Check sheet for the drawn part. Datum: minimum x, y, z corner. Units: mm. A direction names the side the tool comes from. Give positions to 0.01 mm unless a question says otherwise; leave off trailing zeros. Order: outer loops, then holes, each group sorted by start corner. A loop starts at its lowest first (then second) coordinate and runs counter-clockwise, first axis right, second up. Notation, with made-up numbers: M 23,60 L 73,60 A24 ccw 73,73 Z; hole C 14.5,-32 d4. An arc over 180 degrees is marked long. Answer as CSV lines item,"result". Start each with the question number.
Q1. Section check A-A, the plane x = 36. Record the boundary of the cut face in (y, z), then the cut area to 3 significant figures.
Q2. Go/stop test with flat-tipped pins: pin 1 (5 mm diameter, centred on x = 14.5, y = 16.5, fed in from -Z); pin 2 (4 mm diameter, centred on x = 26, z = 2, fed in from +Y); pin 3 (8 mm diameter, centred on x = 38, y = 40, fed in from -Z); pin 4 (6 mm diameter, centred on y = 15.5, z = 26, fed in from -X). Record where each tip stops, or that it passes through.
Q3. Set-up check for the marked faces 1, 2, 3, 4 and 5: record each of +Z, -Z, +X, -X, +Y, -Y from which the full face is reachable in a straight line by a thin tool's end or side.
Q4. Section check C-C, the plane y = 25. Record the boundary of the cut face in (x, z).
Q5. Mould release check, pull along Z, two halves, no side actions. Record for the marked faces 6, 7, 8 and 9: +Z half, -Z half, draft (parallel to the pull), parting line (faces both ways), or undercut.
Q6. Thickness scan on line 1 (X direction, y = 5.75, z = 23); line 2 (Y direction, x = 36, z = 10); line 3 (X direction, y = 42.5, z = 17). Record the ranges inside material, lowest first.
Q7. Section check B-B, the plane z = 22. Record the boundary of the cut face in (x, y).
Q8. Section check D-D, the plane z = 15. Record the boundary of the cut face in (x, y), then the cut area to 3 significant figures.
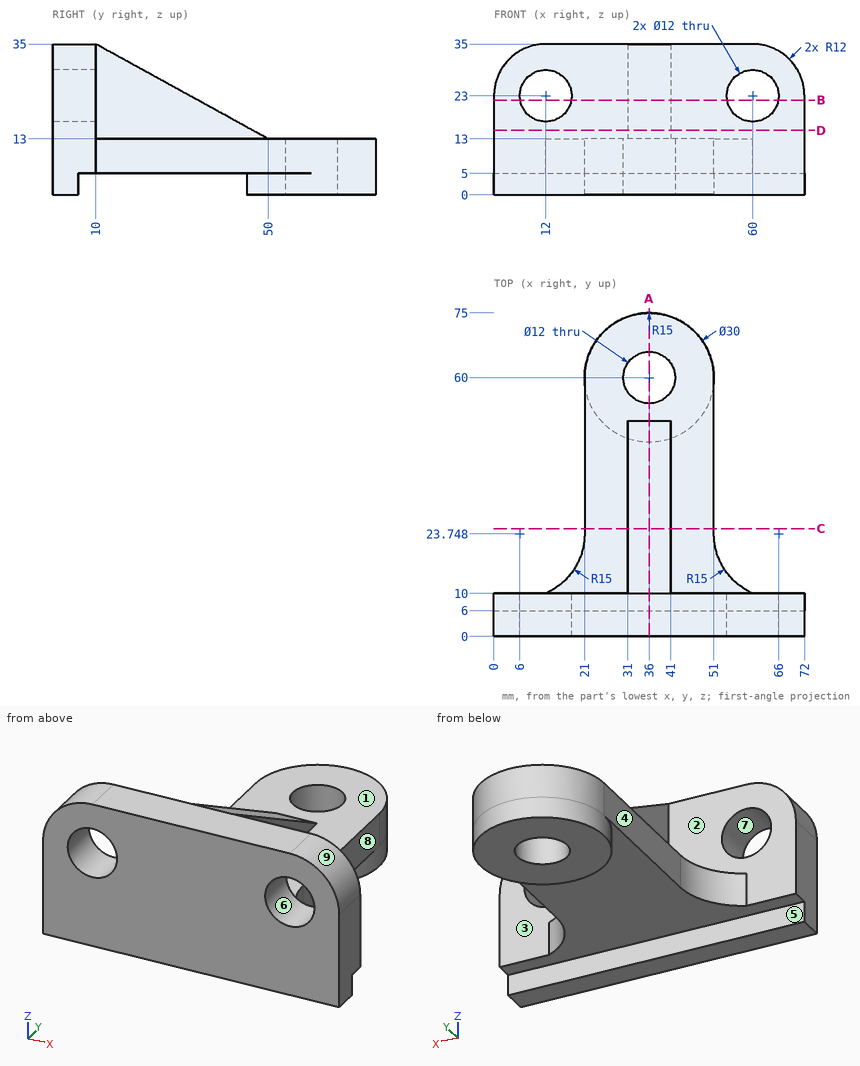
Answer block:
1,outline,"M 0,0 L 6,0 L 6,5 L 45,5 L 45,0 L 54,0 L 54,13 L 50,13 L 10,35 L 0,35 Z; M 66,0 L 75,0 L 75,13 L 66,13 Z"
1,area,"1,280 mm2"
2,pin 1,"passes through"
2,pin 2,"stops at y = 72.69"
2,pin 3,"stops at z = 5"
2,pin 4,"stops at x = 31"
3,face 1,"+Z, +Y"
3,face 2,"+Z, -X, +Y"
3,face 3,"+Z, +X, +Y"
3,face 4,"+Z, -Z, -X, +Y"
3,face 5,"-Z, +X, -X"
4,outline,"M 21,5 L 51,5 L 51,13 L 41,13 L 41,26.75 L 31,26.75 L 31,13 L 21,13 Z"
5,face 6,"undercut"
5,face 7,"undercut"
5,face 8,"draft"
5,face 9,"+Z half"
6,line 1,"x = 0 to 6, 18 to 54, 66 to 72"
6,line 2,"y = 0 to 54, 66 to 75"
6,line 3,"x = 31 to 41"
7,outline,"M 0,0 L 6.08,0 L 6.08,10 L 0,10 Z; M 17.92,0 L 54.08,0 L 54.08,10 L 41,10 L 41,33.64 L 31,33.64 L 31,10 L 17.92,10 Z; M 65.92,0 L 72,0 L 72,10 L 65.92,10 Z"
8,outline,"M 0,0 L 72,0 L 72,10 L 41,10 L 41,46.36 L 31,46.36 L 31,10 L 0,10 Z"
8,area,"1,080 mm2"
